Input: part model. Units: mm. Frame: model coordinates. A direction names the side the tool comes from. Coordinates: 2 decimals unless noted, no trailing zeros. Order: outer loops, then holes, each group sorted by start corner. A loop starts at its lowest first (then second) coordinate and runs counter-clockwise, first axis right, second up. Notation, with made-up numbers: (1, 67) -> (26, 67) arc R18 ccw to (26, 77) -> close; hole circle Ø3 at (75.25, 29.25). An arc over 180 degrees is marked (long way). One line per question, with ' | ' between items.
```python
from build123d import *

# Parameters (mm, degrees)
CROQUIS2_W              = 170
CROQUIS2_H              = 110
SALIENTE_EXTRUIR1_DEPTH = 4
CROQUIS3_W              = 170
CROQUIS3_H              = 110
CROQUIS3_W_2            = 155
CROQUIS3_H_2            = 95
SALIENTE_EXTRUIR2_DEPTH = 20
CROQUIS4_W              = 70
CROQUIS4_H              = 15
CORTAR_EXTRUIR1_DEPTH   = 20
CROQUIS5_W              = 77.5
CROQUIS5_H              = 20
CORTAR_EXTRUIR2_DEPTH   = 20


with BuildPart() as part:
    # Croquis2 → Saliente-Extruir1 (new body)
    with BuildSketch(Plane(origin=(0, 0, 0), x_dir=(1, 0, 0), z_dir=(0, 1, 0))):
        Rectangle(CROQUIS2_W, CROQUIS2_H)
    extrude(amount=SALIENTE_EXTRUIR1_DEPTH)

    # Croquis3 → Saliente-Extruir2 (add)
    with BuildSketch(Plane(origin=(0, 4, 0), x_dir=(1, 0, 0), z_dir=(0, 1, 0))):
        Rectangle(CROQUIS3_W, CROQUIS3_H)
        Rectangle(CROQUIS3_W_2, CROQUIS3_H_2, mode=Mode.SUBTRACT)
    extrude(amount=SALIENTE_EXTRUIR2_DEPTH)

    # Croquis4 → Cortar-Extruir1 (cut)
    with BuildSketch(Plane(origin=(-77.5, 0, 0), x_dir=(0, 0, -1), z_dir=(1, 0, 0))):
        with Locations((2.5, 11.5)):
            Rectangle(CROQUIS4_W, CROQUIS4_H)
    extrude(amount=-CORTAR_EXTRUIR1_DEPTH, mode=Mode.SUBTRACT)

    # Croquis5 → Cortar-Extruir2 (cut)
    with BuildSketch(Plane.XY.offset(-47.5)):
        with Locations((38.75, 14)):
            Rectangle(CROQUIS5_W, CROQUIS5_H)
    extrude(amount=-CORTAR_EXTRUIR2_DEPTH, mode=Mode.SUBTRACT)


solid = part.part
```
1. Pin query (flat end, axial travel): pin 1 Ø1 at (y, z) = (18, -8.5) entering from -X; pin 2 Ø12 at (x, y) = (13, 18) entering from -Z. Return the tip coordinate at first contact, or that it passes through.
Recorded:
pin 1: stops at x = 77.5 | pin 2: stops at z = 47.5
2. Cut plane D-D, the plane z = 34.5. Return loops of the section in (x, y).
Recorded:
outline: (-85, 0) -> (85, 0) -> (85, 24) -> (77.5, 24) -> (77.5, 4) -> (-77.5, 4) -> (-77.5, 24) -> (-85, 24) -> close
3. Cut plane B-B, the plane y = 15. Return loops of the section in (x, z).
Recorded:
outline: (-85, -55) -> (0, -55) -> (0, -47.5) -> (-77.5, -47.5) -> (-77.5, -37.5) -> (-85, -37.5) -> close; (-85, 32.5) -> (-77.5, 32.5) -> (-77.5, 47.5) -> (77.5, 47.5) -> (77.5, -55) -> (85, -55) -> (85, 55) -> (-85, 55) -> close
4. Cut plane A-A, the plane z = 14.5. Return loops of the section in (x, y).
Recorded:
outline: (-85, 0) -> (85, 0) -> (85, 24) -> (77.5, 24) -> (77.5, 4) -> (-85, 4) -> close; (-85, 19) -> (-77.5, 19) -> (-77.5, 24) -> (-85, 24) -> close
5. Ray query, line 1 (X direction, y = 21.5, z = 29.5); line 2 (Z direction, x = -46.5, y = 15.25); line 3 (X direction, y = 10.25, z = -33). Return the intervals inside material, ascending. Write a range as [from, to].
Recorded:
line 1: x = [-85, -77.5], [77.5, 85] | line 2: z = [-55, -47.5], [47.5, 55] | line 3: x = [77.5, 85]
6. Cut plane C-C, the plane x = -51. Return loops of the section in (y, z), and give its area (3 significant figures).
Recorded:
outline: (0, -55) -> (24, -55) -> (24, -47.5) -> (4, -47.5) -> (4, 47.5) -> (24, 47.5) -> (24, 55) -> (0, 55) -> close | area: 740 mm^2
7. Access query for faces 4 (the face through (-77.5, 21, 1)), 5 (the face through (-81, 19, -2)), 6 (the face through (77.5, 14, -3)), 7 (the face through (-85, 3.8, 0.8)). Directions: +Z, -Z, +X, -X, +Y, -Y. A direction counts if a zero-diameter tool reaches every point of the face in a straight line with its end or side. Return the directions, or none.
Recorded:
face 4: +Y | face 5: -X | face 6: -Z, +Y | face 7: +Z, -Z, -X, +Y, -Y
8. Mould query, pull axis X, two halves, no side actions, for faces 1 (the face through (0, 14, -51)), 2 (the face through (-81, 11, -37.5)), 3 (the face through (85, 12, 1)). Classes: released by +X, released by -X, zero draft, split by the parting line, or undercut.
Recorded:
face 1: undercut | face 2: zero draft | face 3: released by +X
